Source: CAD feature listing. Evaluate the final solid. Frame: model axes, mm. Round coordinates to 2 decimals unless told otherwise and drop trailing zeros. Write each loop counter-clockwise with the first axis right and the second up, starting at its lowest first coordinate (ties: lowest second). Pieces come first, ordered by that corner, then holes.
```python
from build123d import *

# Parameters (mm, degrees)
CYLINDER066_R     = 7
CYLINDER066_DEPTH = 5
CYLINDER067_R     = 15
CYLINDER067_DEPTH = 5
FILLET006_R       = 1
FILLET007_R       = 1


with BuildPart() as cylindre062:
    # Cylinder066 → Cylinder066 (new body)
    with BuildSketch(Plane(origin=(0, -4, -107), x_dir=(1, 0, 0), z_dir=(0, -1, 0))):
        Circle(CYLINDER066_R)
    extrude(amount=CYLINDER066_DEPTH)


with BuildPart() as fillet007:
    # Cylinder067 → Cylinder067 (new body)
    with BuildSketch(Plane(origin=(0, -4, -107), x_dir=(1, 0, 0), z_dir=(0, -1, 0))):
        Circle(CYLINDER067_R)
    extrude(amount=CYLINDER067_DEPTH)

    # Cut040: cut Cylindre062
    add(cylindre062.part, mode=Mode.SUBTRACT)

    # Fillet006
    fillet006_edges = [fillet007.edges().sort_by_distance(p)[0] for p in [
        (-15, -4, -107),
    ]]
    fillet(fillet006_edges, radius=FILLET006_R)

    # Fillet007
    fillet007_edges = [fillet007.edges().sort_by_distance(p)[0] for p in [
        (-15, -9, -107),
    ]]
    fillet(fillet007_edges, radius=FILLET007_R)


solid = fillet007.part
```
Q1. Section query C-C, the plane y = -7.5. Output: boundary loops of the cut face in (x, z), and give its area (3 significant figures).
Q2. Line query: line 1 (Z direction, x = 0, y = -7.4); line 2 (X direction, y = -7.2, z = -111.25); line 3 (X direction, y = -7.25, z = -104.25). Output: solid intervals per line, ascending.
Q3. Section query A-A, the plane x = 0. Output: boundary loops of the cut face in (y, z), and give its area (3 significant figures).
Q4. Section query B-B, the plane z = -107. Output: boundary loops of the cut face in (x, y), and give its area (3 significant figures).
Q5. Mould query, pull axis X, two halves, no side actions, for faces 1 (the face through (-0.91, -6.46, -100.06)), 2 (the face through (-3.252, -6.479, -121.643)), 3 (the face through (-6.4, -4, -103.7)). Classes: pulls with the +X half, pulls with the -X half, needs draft (parallel to the pull), parting line crosses it, or undercut.
Q6. Pin query (flat end, axial travel): P1, Ø1, axis at y = -5, z = -103, coming from the +X side; P2, Ø1, axis at x = -6, y = -7, coming from the -Z side; P3, Ø2, axis at x = 7.5, y = -7, coming from the +Z side. Return the tip coordinate at first contact, or that it passes through.
Filled in:
1. outline: circle Ø30 at (0, -107); hole circle Ø14 at (0, -107)
1. area: 553 mm2
2. line 1: z = -122 to -114, -100 to -92
2. line 2: x = -14.39 to -5.56, 5.56 to 14.39
2. line 3: x = -14.75 to -6.44, 6.44 to 14.75
3. outline: (-9, -121) arc R1 ccw to (-8, -122) - (-5, -122) arc R1 ccw to (-4, -121) - (-4, -114) - (-9, -114) - close; (-9, -100) - (-4, -100) - (-4, -93) arc R1 ccw to (-5, -92) - (-8, -92) arc R1 ccw to (-9, -93) - close
3. area: 79.1 mm2
4. outline: (-15, -8) arc R1 ccw to (-14, -9) - (-7, -9) - (-7, -4) - (-14, -4) arc R1 ccw to (-15, -5) - close; (7, -9) - (14, -9) arc R1 ccw to (15, -8) - (15, -5) arc R1 ccw to (14, -4) - (7, -4) - close
4. area: 79.1 mm2
5. face 1: undercut
5. face 2: parting line crosses it
5. face 3: needs draft
6. P1: stops at x = 14.59
6. P2: stops at z = -120.96
6. P3: stops at z = -93.48
